Input: part model. Units: mm. Frame: model coordinates. A direction names the side the tool comes from. Round coordinates to 2 decimals unless told otherwise and drop trailing zeros. Loops run counter-clockwise (first coordinate to the right, second up) from the corner with the lowest first, then second, coordinate; pieces in that order, holes last. Notation, with made-up numbers: (-22, 69) - (-4, 69) arc R21 cw to (-4, 86) - close; hole circle Ø8 at (-36, 81.5). An arc over 180 degrees is marked (long way). Write each question's results on one line, items separated by ' | '.
from build123d import *

# Parameters (mm, degrees)
SKETCH1_W           = 27.5
SKETCH1_H           = 47
BOSS_EXTRUDE1_DEPTH = 25
SKETCH2_R           = 1.5
BOSS_EXTRUDE2_DEPTH = 2.25
CHAMFER1_SIZE       = 1
FILLET1_R           = 0.5


with BuildPart() as part:
    # Sketch1 → Boss-Extrude1 (new body)
    with BuildSketch(Plane(origin=(0, 0, 0), x_dir=(1, 0, 0), z_dir=(0, 1, 0))):
        with Locations((13.75, 23.5)):
            Rectangle(SKETCH1_W, SKETCH1_H)
    extrude(amount=BOSS_EXTRUDE1_DEPTH)

    # Sketch2 → Boss-Extrude2 (add)
    with BuildSketch(Plane(origin=(0, 25, 0), x_dir=(1, 0, 0), z_dir=(0, 1, 0))):
        Polygon((0, 53.25), (27.5, 53.25), (38.25, 23.5), (27.5, -6.25), (0, -6.25), (-10.75, 23.5), align=None)
        with Locations((-6, 23.5)):
            Circle(SKETCH2_R, mode=Mode.SUBTRACT)
        with Locations((33.5, 23.5)):
            Circle(SKETCH2_R, mode=Mode.SUBTRACT)
    extrude(amount=BOSS_EXTRUDE2_DEPTH)

    # Chamfer1
    chamfer1_edges = [part.edges().sort_by_distance(p)[0] for p in [
        (-7.5, 27.25, -23.5),
        (32, 27.25, -23.5),
    ]]
    chamfer(chamfer1_edges, length=CHAMFER1_SIZE)

    # Fillet1
    fillet1_edges = [part.edges().sort_by_distance(p)[0] for p in [
        (-5.375, 27.25, -38.375),
        (-5.375, 27.25, -8.625),
        (13.75, 27.25, 6.25),
        (32.875, 27.25, -8.625),
        (32.875, 27.25, -38.375),
        (13.75, 27.25, -53.25),
        (0, 26.125, -53.25),
        (-10.75, 26.125, -23.5),
        (0, 26.125, 6.25),
        (27.5, 26.125, 6.25),
        (38.25, 26.125, -23.5),
        (27.5, 26.125, -53.25),
        (31, 27.25, -23.5),
        (-8.5, 27.25, -23.5),
        (0, 12.5, -47),
        (27.5, 12.5, -47),
        (27.5, 12.5, 0),
        (0, 12.5, 0),
    ]]
    fillet(fillet1_edges, radius=FILLET1_R)


solid = part.part
1. Set-up query: faces 1 (the flat face through (-1, 25, -21)), 2 (the flat face through (0, 12, -23)), 3 (the flat face through (14, 26, -53.25)). Return all of +Z, -Z, +X, -X, +Y, -Y with unobstructed straight access to the full face (end or side cutting, diameter ignored); none if empty.
Answer:
face 1: -Y | face 2: +Z, -Z, -X, -Y | face 3: -Z, +X, -X, +Y, -Y
2. Section query B-B, the plane y = 22. Output: boundary loops of the cut face in (x, z), plus the area to 3 significant figures.
Answer:
outline: (0, -46.5) arc R0.5 ccw to (0.5, -47) - (27, -47) arc R0.5 ccw to (27.5, -46.5) - (27.5, -0.5) arc R0.5 ccw to (27, 0) - (0.5, 0) arc R0.5 ccw to (0, -0.5) - close | area: 1,290 mm^2
3. Section query A-A, the plane x = 20. Output: boundary loops of the cut face in (y, z).
Answer:
outline: (0, -47) - (25, -47) - (25, -53.25) - (26.75, -53.25) arc R0.5 ccw to (27.25, -52.75) - (27.25, 5.75) arc R0.5 ccw to (26.75, 6.25) - (25, 6.25) - (25, 0) - (0, 0) - close
4. Contact query for flat-ended pins moving along their axis: pin 1 (1.5 mm diameter, centred on y = 8, z = -9, fed in from -X); pin 2 (1 mm diameter, centred on x = 18, y = 17.5, fed in from -Z); pin 3 (10 mm diameter, centred on x = 0.5, y = 9, fed in from +Z). Output: stop coordinate, or through.
Answer:
pin 1: x = 0 | pin 2: z = -47 | pin 3: z = 0
5. Mould query, pull axis Z, two halves, no side actions, for faces 4 (the flat face through (14, 12, -47)), 5 (the flat face through (14, 26, 6.25)), 6 (the cylindrical face through (32.39, 25.62, -24.51)), 7 (the flat face through (14, 0, -24)). Classes: pulls with the +Z half, pulls with the -Z half, needs draft (parallel to the pull), parting line crosses it, or undercut.
Answer:
face 4: pulls with the -Z half | face 5: pulls with the +Z half | face 6: undercut | face 7: needs draft
6. Line query: line 1 (Z direction, x = 7.5, y = 19.75); line 2 (Y direction, x = 29, z = -23); line 3 (X direction, y = 24, z = -27.5). Output: solid intervals per line, ascending. Write a range as [from, to].
Answer:
line 1: [-47, 0] | line 2: [25, 27.25] | line 3: [0, 27.5]
